Drawing for the job (mm, zero at the part's lowest x, y, z). Coordinates: 2 decimals unless noted, no trailing zeros. Write each loop counter-clockwise with the first axis right and the second up, starting at its lowest first coordinate (ties: lowest second). Pieces come first, ordered by that corner, then holes. Notation, with made-up numbers: M -36,16 L -14,16 A23 cw -14,55 Z; hole C 14.25,40 d5. An arc over 180 degrees is marked long. Use a Markdown table: item, result. Add a question column.
Q1. Slice it at B-B on y = 6.5. Write the cut outline in (x, z), then the cut area to 3 significant figures.
Q2. Slice it at C-C on z = 55.5. Write the cut outline in (x, y), then the cut area to 3 significant figures.
Q3. Mould opens along X. For the marked faces 1, 2, 3 and 4 say: released by +X, released by -X, zero draft, split by the parting line, or undercut.
Q4. Slice it at D-D on z = 80. Write the cut outline in (x, y), then the cut area to 3 significant figures.
Q5. Slice it at A-A on x = 54. Write the cut outline in (y, z), then the cut area to 3 significant figures.
Q6. Wall check: L1, parallel to Z at x = 57.5, y = 16.75; L2, parallel to X at y = 7.5, z = 54; L3, parallel to Z at x = 56.5, y = 8.75. Give the ranges that are in metal, low to high. Write a range as from..to.
Q7. Pin check, flat tips, straight feed: pin 1 Ø1.1 at (x, y) = (41, 6) entering from -Z; pin 2 Ø8 at (x, y) = (22.5, 9.5) entering from -Z; pin 3 Ø1.5 at (x, y) = (71, 3) entering from +Z. Stop position of each tip, or through.
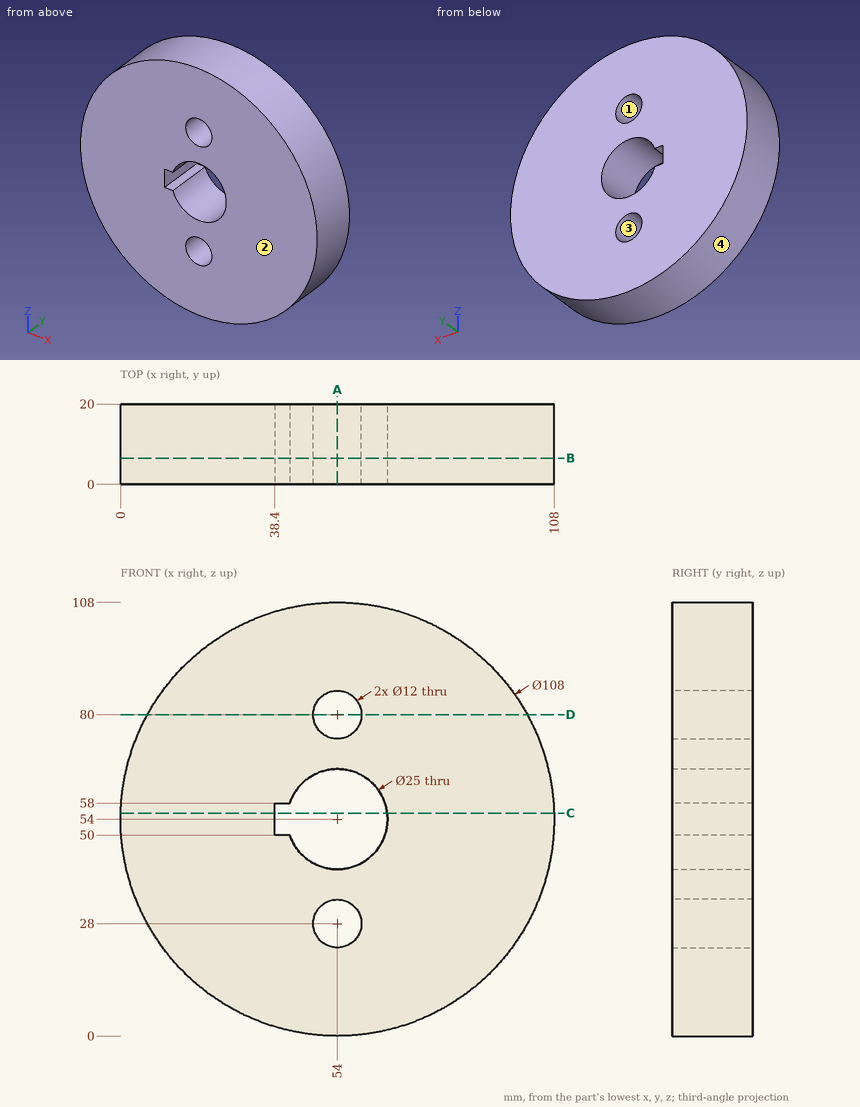
Recorded:
| question | item | result |
|---|---|---|
| 1 | outline | C 54,54 d108; hole M 38.4,50 L 42.16,50 A12.5 ccw long 42.16,58 L 38.4,58 Z; hole C 54,28 d12; hole C 54,80 d12 |
| 1 | area | 8,420 mm² |
| 2 | outline | M 0.02,0 L 38.4,0 L 38.4,20 L 0.02,20 Z; M 66.41,0 L 107.98,0 L 107.98,20 L 66.41,20 Z |
| 2 | area | 1,600 mm² |
| 3 | face 1 | undercut |
| 3 | face 2 | zero draft |
| 3 | face 3 | undercut |
| 3 | face 4 | split by the parting line |
| 4 | outline | M 6.67,0 L 48,0 L 48,20 L 6.67,20 Z; M 60,0 L 101.33,0 L 101.33,20 L 60,20 Z |
| 4 | area | 1,650 mm² |
| 5 | outline | M 0,0 L 20,0 L 20,22 L 0,22 Z; M 0,34 L 20,34 L 20,41.5 L 0,41.5 Z; M 0,66.5 L 20,66.5 L 20,74 L 0,74 Z; M 0,86 L 20,86 L 20,108 L 0,108 Z |
| 5 | area | 1,180 mm² |
| 6 | L1 | 0.11..23.13, 32.87..42, 66..75.13, 84.87..107.89 |
| 6 | L2 | 0..38.4, 66.5..108 |
| 6 | L3 | 0.06..22.55, 33.45..41.75, 66.25..74.55, 85.45..107.94 |
| 7 | pin 1 | z = 1.45 |
| 7 | pin 2 | z = 7.53 |
| 7 | pin 3 | z = 105.5 |
